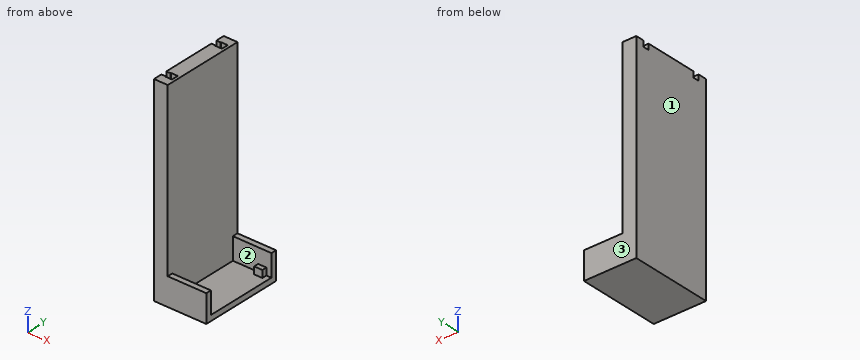
```python
from build123d import *

# Parameters (mm, degrees)
F1_DEPTH  = 76.2
F3_DEPTH  = 25.4
F4_DEPTH  = 5.08
F5_W      = 7.62
F5_H      = 4.3815
F6_DEPTH  = 11.684
F7_W      = 6.35
F7_H      = 6.35
F8_DEPTH  = 55.88
F9_W      = 5.334
F9_H      = 5.334
F10_DEPTH = 5.08


# Not quite as in the source:
# - a feature names something its author has since deleted; it is built from what else it names


with BuildPart() as f1:
    # F0 (on Front) → F1 (new body)
    with BuildSketch(Plane.XZ):
        Polygon((0, 0), (12.7, 0), (12.7, 5.4184001555), (12.7, 23.5612627981), (12.7, 183.226400471), (0, 183.226400471), align=None)
    extrude(amount=F1_DEPTH)

    # F2 (on Top) → F3 (join)
    with BuildSketch(Plane.XY):
        Polygon((43.18, 0), (0, 0), (0, -5.0670392811), (48.26, -5.0670392811), (48.26, 0), align=None)
        Polygon((27.7881938964, -71.1809098721), (0, -71.1809098721), (0, -76.2), (30.48, -76.2), (48.26, -76.2), (48.26, -71.1809098721), (35.56, -71.1809098721), align=None)
    extrude(amount=F3_DEPTH)

    # F2 (on Top) → F4 (join)
    with BuildSketch(Plane.XY):
        Polygon((43.18, 0), (0, 0), (0, -5.0670392811), (48.26, -5.0670392811), (48.26, 0), align=None)
        Polygon((48.26, -5.0670392811), (0, -5.0670392811), (0, -71.1809098721), (27.7881938964, -71.1809098721), (35.56, -71.1809098721), (48.26, -71.1809098721), align=None)
    extrude(amount=F4_DEPTH)

    # F5 (on Top) → F6 (join)
    with BuildSketch(Plane.XY):
        with Locations((39.8590039933, -7.2577892811)):
            Rectangle(F5_W, F5_H)
        with Locations((39.8590039933, -68.9901598721)):
            Rectangle(F5_W, F5_H)
    extrude(amount=F6_DEPTH)

    # F7 (on face) → F8 (cut)
    with BuildSketch(Plane.XY.offset(183.226400471)):
        with Locations((6.985, -10.795)):
            Rectangle(F7_W, F7_H)
        with Locations((6.985, -65.405)):
            Rectangle(F7_W, F7_H)
    extrude(amount=-F8_DEPTH, mode=Mode.SUBTRACT)

    # F9 (on Right) → F10 (cut)
    with BuildSketch(Plane.YZ):
        with Locations((-65.405, 180.559400471)):
            Rectangle(F9_W, F9_H)
        with Locations((-10.795, 180.559400471)):
            Rectangle(F9_W, F9_H)
    extrude(amount=F10_DEPTH, mode=Mode.SUBTRACT)


solid = f1.part
```
Read the model definition and answer for the solid it produces. Units are mm, in the model's axes. Face numbers are marked on the shaded views. Coordinates: 2 decimals unless noted, no trailing zeros. Write each loop counter-clockwise with the first axis right and the second up, starting at its lowest first coordinate (ties: lowest second). Pieces come first, ordered by that corner, then holes. Notation, with made-up numbers: (80, -29) -> (122, -29) arc R25 ccw to (122, -11) -> close; hole circle Ø4 at (83, 49.25). An arc over 180 degrees is marked (long way). Return JSON: item names as keys, results as strings.
1. A cutting plane is placed at A-A (x = 20.5). Determine the outline of the cut face in (y, z), and give its area (3 significant figures).
Found:
{"outline": "(-76.2, 0) -> (0, 0) -> (0, 25.4) -> (-5.07, 25.4) -> (-5.07, 5.08) -> (-71.18, 5.08) -> (-71.18, 25.4) -> (-76.2, 25.4) -> close", "area": "592 mm2"}
2. A cutting plane is placed at B-B (z = 161.5). Determine the outline of the cut face in (x, y), and give its area (3 significant figures).
Found:
{"outline": "(0, -76.2) -> (12.7, -76.2) -> (12.7, 0) -> (0, 0) -> close; hole (3.81, -68.58) -> (10.16, -68.58) -> (10.16, -62.23) -> (3.81, -62.23) -> close; hole (3.81, -13.97) -> (10.16, -13.97) -> (10.16, -7.62) -> (3.81, -7.62) -> close", "area": "887 mm2"}
3. Find the intervals of material crossed by line 1 along Z through (x, y) = (46, -53); line 2 along X through (y, z) = (-8, 64.5), in increasing order. Write a range as from..to.
Found:
{"line 1": "0..5.08", "line 2": "0..12.7"}
4. A cutting plane is placed at C-C (y = -21.5). Determine the outline of the cut face in (x, z), and give its area (3 significant figures).
Found:
{"outline": "(0, 0) -> (48.26, 0) -> (48.26, 5.08) -> (12.7, 5.08) -> (12.7, 183.23) -> (0, 183.23) -> close", "area": "2,510 mm2"}
5. Determine the mould class of the marked faces 1, 2 and 3 for opening direction Y: pulls with the +Y half, pulls with the -Y half, needs draft (parallel to the pull), parting line crosses it, or undercut.
Found:
{"face 1": "needs draft", "face 2": "undercut", "face 3": "pulls with the +Y half"}
6. Each of these flat-tipped pins is pushed along its axis until it touches: P1, Ø3, axis at y = -56, z = 116, coming from the +X side; P2, Ø1.3, axis at y = -6.5, z = 8, coming from the +X side; P3, Ø5.5, axis at x = 33.5, y = -72.5, coming from the +Z side. Where does it stop, or does it pass through?
Found:
{"P1": "x = 12.7", "P2": "x = 43.67", "P3": "z = 25.4"}
7. A cutting plane is placed at D-D (z = 52.5). Determine the outline of the cut face in (x, y).
Found:
{"outline": "(0, -76.2) -> (12.7, -76.2) -> (12.7, 0) -> (0, 0) -> close"}
